Autodesk Inventor part; units mm, degrees
ref_plane "YZ Plane" through (0, 0, 0) normal (1, 0, 0) x (0, 1, 0)
ref_plane "XZ Plane" through (0, 0, 0) normal (0, 1, 0) x (-1, 0, 0)
ref_plane "XY Plane" through (0, 0, 0) normal (0, 0, 1) x (1, 0, 0)
sketch "Sketch1" plane through (0, 0, 0) normal (0, 0, 1) x (1, 0, 0)
  line L0 (-750, 0) -> (750, 0) construction
  line L1 (750, 0) -> (750, -2700) construction
  line L2 (750, -2700) -> (-750, -2700) construction
  line L3 (-750, -2700) -> (-750, 0) construction
  line L4 (800, 50) -> (-800, 50) construction
  line L5 (-800, 50) -> (-800, -2750) construction
  line L6 (-800, -2750) -> (800, -2750) construction
  line L7 (800, -2750) -> (800, 50) construction
  line L8 (-850, 100) -> (850, 100) construction
  line L9 (850, 100) -> (850, -2800) construction
  line L10 (850, -2800) -> (-850, -2800) construction
  line L11 (-850, -2800) -> (-850, 100) construction
  arc A0 (750, 0) -> (742.111681, 1.050817) centre (0, -5600) ccw construction
  line L12 (-750, -2100) -> (750, -2100) construction
  line L13 (115.485997, -2697.8227) -> (750, -2100) construction
  arc A1 (750, -2100) -> (750, 0) centre (-10250, -1050) ccw construction
  arc A2 (110, -2700) -> (115.485997, -2697.8227) centre (110, -2692) ccw construction
  arc A3 (742.111681, 1.050817) -> (0, 50) centre (0, -5600) ccw
  line L14 (0, 100) -> (0, 50) construction
  line L15 (0, -2700) -> (0, -2697) construction
  line L16 (0, 47) -> (0, 0) construction
  line L17 (0, 50) -> (0, 47) construction
  line L18 (750.763103, -8.025362) -> (770.411716, -241.9)
  arc A4 (750.763103, -8.025362) -> (742.111681, 1.050817) centre (740.798209, -8.862547) ccw
  point P0 (0, -2750)
  dimension "d54" = 1500
  dimension "d55" = 2700
  dimension "d58" = 2100
  dimension "d83" = 8
  dimension "d113" = 50
  dimension "d114" = 50
  dimension "d115" = 3
  dimension "d121" = 10
  dimension "d122" = 241.9
  dimension "d124" = 94.8023
contour flange "Contour Flange2" sketch "Sketch1" thickness 3 bend radius 5 width 950 along (0, 0, 1) mid plane no both sides no wall seen from (760.58741, -124.962681, 0) lies toward (-0.9964894, -0.0837185, 0) curves L18 A4 A3
bend "Bend2"
corner "Corner2"
mirror "Mirror2" about plane through (0, 0, 0) normal (1, 0, 0)
sketch "Sketch2" plane through (747.773635, -8.276518, 0) normal (-0.9964894, -0.0837185, 0) x (0, 0, 1)
  line L0 (931.668513, -217.277497) -> (809.542302, -217.277497) construction
  line L1 (809.542302, -217.277497) -> (809.542302, -193.633612) construction
  line L2 (809.542302, -193.633612) -> (931.668513, -193.633612) construction
  line L3 (931.668513, -193.633612) -> (931.668513, -217.277497) construction
  point P0 (0, 70.849954)
mark "Mark1"
equation "\"d36\" = Thickness"
equation "\"d37\" = BendReliefWidth"
equation "\"d38\" = BendReliefDepth"
equation "\"d39\" = MinimumRemnant"
equation "\"d40\" = TransitionRadius"
equation "\"d42\" = BendRadius"
equation "\"d44\" = CornerReliefSize"
equation "\"d45\" = GapSize"
equation "\"d46\" = JacobiRadiusSize"
equation "\"BendReliefWidth\" = Thickness"
equation "\"BendReliefDepth\" = 0.5 * Thickness"
equation "\"CornerReliefSize\" = 4 * Thickness"
equation "\"MinimumRemnant\" = 2 * Thickness"
equation "\"GapSize\" = Thickness"
properties part number "MSC 208 SHEET BACK START" material "Stainless Steel AISI 304"
Check sheet for the modelled part. Datum: model origin and axes. Units: mm. Give positions to 0.01 mm unless a question says otherwise; leave off trailing zeros. Write each loop counter-clockwise with the first axis right and the second up, starting at its lowest first coordinate (ties: lowest second). Pieces come first, ordered by that corner, then holes. Notation, with made-up numbers: M 32,34 L 63,34 A24 cw 63,62 Z; hole C 0,52.25 d10. An arc over 180 degrees is marked long. Use one line per item in the form item = value.
(1) Section check D-D on x = -265.5. Record the boundary of the cut face in (y, z), plus the area to 3 significant figures.
Answer block:
outline = M 40.76,0 L 43.76,0 L 43.76,950 L 40.76,950 Z
area = 2,850 mm2
(2) Material ranges on line 1 along X through (y, z) = (-46, 668); line 2 along X through (y, z) = (-189.5, 651.5); line 3 along Y through (x, z) = (27.5, 533.5), recorded low to high.
Answer block:
line_1 = -753.95 to -750.94, 750.94 to 753.95
line_2 = -766.01 to -763, 763 to 766.01
line_3 = 46.93 to 49.93
(3) Draft check along X on faces 1 (the flat face through (760.45, -123.33, 468.35)), 2 (the flat face through (-757.735, -126.851, 468.35)), 3 (the flat face through (-760.725, -126.6, 468.35)). Enter one of: pulls with the +X half, pulls with the -X half, needs draft (parallel to the pull), parting line crosses it, or undercut.
Answer block:
face_1 = pulls with the +X half
face_2 = undercut
face_3 = pulls with the -X half
(4) Section check A-A on y = -197.5. Record the boundary of the cut face in (x, z).
Answer block:
outline = M -766.68,0 L -763.67,0 L -763.67,950 L -766.68,950 Z; M 763.67,0 L 766.68,0 L 766.68,950 L 763.67,950 Z
(5) Section check C-C on x = 35.5. Record the boundary of the cut face in (y, z).
Answer block:
outline = M 46.89,0 L 49.89,0 L 49.89,950 L 46.89,950 Z
(6) Depth check by flat-ended pin: P1, Ø4, axis at x = 595.5, z = 249.5, coming from the +Y side; P2, Ø1.5, axis at y = -49.5, z = 585, coming from the -X side; P3, Ø6, axis at y = -115.5, z = 797, coming from the +X side. Enter the tip coordinate at first touch or a pass-through.
Answer block:
P1 = 18.74
P2 = -754.31
P3 = 760.04
(7) Section check B-B on z = 255. Record the boundary of the cut face in (x, y), plus the area to 3 significant figures.
Answer block:
outline = M -770.41,-241.9 L -767.42,-242.15 L -747.77,-8.28 A7 cw -741.72,-1.92 A5647 cw 0,47 A5647 cw 741.72,-1.92 A7 cw 747.77,-8.28 L 767.42,-242.15 L 770.41,-241.9 L 750.76,-8.03 A10 ccw 742.11,1.05 A5650 ccw 0,50 A5650 ccw -742.11,1.05 A10 ccw -750.76,-8.03 Z
area = 5,940 mm2
